Answer from the drawing. Dimensions are ordinates in mm from the lowest x, y and z of the part. A direction names the side the tool comes from. Round coordinates to 2 decimals unless told otherwise and drop trailing zeros. Write each loop counter-clockwise with the first axis right and the second up, starting at its lowest first coordinate (ties: lowest second). Pieces come first, ordered by that corner, then holes. Notation, with made-up numbers: (-15.75, 6) -> (-0.75, 6) arc R17 ccw to (-0.75, 20) -> close; hole circle Ø11 at (28, -19.5). An arc over 180 degrees is marked (long way). Return JSON: item names as keys, results as strings. Group by question number.
(1) Straight lines are drawn through the part: line 1 (X direction, y = 2, z = 19.75); line 2 (Z direction, x = 28.5, y = 14.5); line 3 (X direction, y = 6.5, z = 14.25). For each, find the intervals that lie inside material, in ascending order.
(2) Given pin 1 (6 mm diameter, centred on x = 18, y = 8, fed in from -Z); pin 2 (0.6 mm diameter, centred on y = 8.5, z = 15, fed in from +X); pin 3 (2 mm diameter, centred on x = 37.5, y = 6.5, fed in from +Z), each flat-ended and moving along its own axis, determine where each tip first touches the part or whether it passes through.
(3) A cutting plane is placed at B-B on z = 15. Give the vertices of the cut face in (x, y), then the cut area to 3 significant figures.
(4) A cutting plane is placed at C-C on x = 24. Give the vertices of the cut face in (y, z), then the cut area to 3 significant figures.
(5) A cutting plane is placed at A-A on y = 15. Give the vertices of the cut face in (x, z).
(6) For the marked faces 1 and 2, determine the directions among +Z, -Z, +X, -X, +Y, -Y from which every point of the face is accessible in a straight line to the end or side of a thin tool.
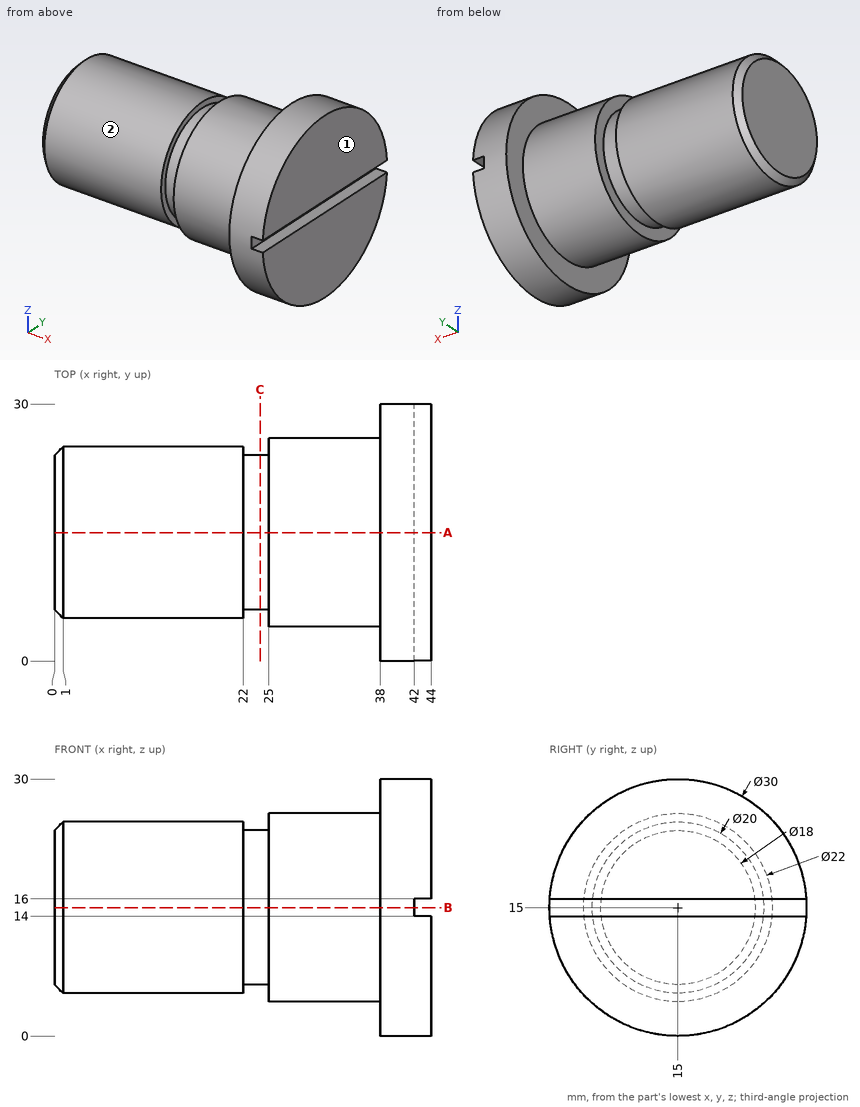
Checks:
{
 "1": {"line 1": "x = 38 to 44", "line 2": "z = 4.01 to 25.99", "line 3": "x = 0 to 42"},
 "2": {"pin 1": "stops at z = 5.83", "pin 2": "stops at x = 42", "pin 3": "stops at z = 27.91"},
 "3": {"outline": "(0, 6) -> (1, 5) -> (22, 5) -> (22, 6) -> (25, 6) -> (25, 4) -> (38, 4) -> (38, 0) -> (42, 0) -> (42, 30) -> (38, 30) -> (38, 26) -> (25, 26) -> (25, 24) -> (22, 24) -> (22, 25) -> (1, 25) -> (0, 24) -> close", "area": "899 mm^2"},
 "4": {"outline": "circle Ø18 at (15, 15)", "area": "254 mm^2"},
 "5": {"outline": "(0, 6) -> (1, 5) -> (22, 5) -> (22, 6) -> (25, 6) -> (25, 4) -> (38, 4) -> (38, 0) -> (44, 0) -> (44, 14) -> (42, 14) -> (42, 16) -> (44, 16) -> (44, 30) -> (38, 30) -> (38, 26) -> (25, 26) -> (25, 24) -> (22, 24) -> (22, 25) -> (1, 25) -> (0, 24) -> close"},
 "6": {"face 1": "+Z, -Z, +X, +Y, -Y", "face 2": "-X"}
}
